```python
from build123d import *

# Parameters (mm, degrees)
SKETCH1_W           = 540
SKETCH1_H           = 540
BOSS_EXTRUDE1_DEPTH = 5
SKETCH2_W           = 20
SKETCH2_H           = 20
CUT_EXTRUDE1_DEPTH  = 5
CHAMFER1_SIZE       = 2
CHAMFER2_SIZE       = 0.5
SKETCH3_W           = 200
SKETCH3_H           = 77.416612185
CUT_EXTRUDE2_DEPTH  = 10
CIRPATTERN1_COUNT   = 4


with BuildPart() as part:
    # Sketch1 → Boss-Extrude1 (new body)
    with BuildSketch(Plane.XY):
        with Locations((270, 270)):
            Rectangle(SKETCH1_W, SKETCH1_H)
    extrude(amount=BOSS_EXTRUDE1_DEPTH)

    # Sketch2 → Cut-Extrude1 (cut)
    with BuildSketch(Plane.XY.offset(5)):
        with Locations((10, 530)):
            Rectangle(SKETCH2_W, SKETCH2_H)
        with Locations((530, 530)):
            Rectangle(SKETCH2_W, SKETCH2_H)
        with Locations((530, 10)):
            Rectangle(SKETCH2_W, SKETCH2_H)
        with Locations((10, 10)):
            Rectangle(SKETCH2_W, SKETCH2_H)
    extrude(amount=-CUT_EXTRUDE1_DEPTH, mode=Mode.SUBTRACT)

    # Chamfer1
    chamfer1_edges = [part.edges().sort_by_distance(p)[0] for p in [
        (0, 20, 2.5),
        (20, 0, 2.5),
        (540, 20, 2.5),
        (520, 0, 2.5),
        (540, 520, 2.5),
        (520, 540, 2.5),
        (0, 520, 2.5),
        (20, 540, 2.5),
    ]]
    chamfer(chamfer1_edges, length=CHAMFER1_SIZE)

    # Chamfer2
    chamfer2_edges = [part.edges().sort_by_distance(p)[0] for p in [
        (11, 20, 0),
        (11, 20, 5),
        (520, 11, 0),
        (520, 11, 5),
        (529, 520, 0),
        (529, 520, 5),
        (20, 529, 0),
        (20, 529, 5),
        (11, 520, 5),
        (11, 520, 0),
        (0, 270, 5),
        (20, 11, 5),
        (270, 0, 5),
        (529, 20, 5),
        (540, 270, 5),
        (520, 529, 5),
        (270, 540, 5),
        (519, 1, 5),
        (539, 21, 5),
        (1, 21, 5),
        (21, 1, 5),
        (539, 519, 5),
        (519, 539, 5),
        (21, 539, 5),
        (1, 519, 5),
        (0, 270, 0),
        (270, 540, 0),
        (520, 529, 0),
        (540, 270, 0),
        (529, 20, 0),
        (270, 0, 0),
        (20, 11, 0),
        (519, 1, 0),
        (539, 21, 0),
        (1, 21, 0),
        (21, 1, 0),
        (539, 519, 0),
        (519, 539, 0),
        (21, 539, 0),
        (1, 519, 0),
    ]]
    chamfer(chamfer2_edges, length=CHAMFER2_SIZE)

    # Sketch3 → Cut-Extrude2 (cut)
    with BuildSketch(Plane.XY.offset(5)):
        with Locations((270, 558.708306093)):
            Rectangle(SKETCH3_W, SKETCH3_H)
    cut_extrude2 = extrude(amount=-CUT_EXTRUDE2_DEPTH, mode=Mode.SUBTRACT)

    # CirPattern1: Cut-Extrude2 ×4 about axis
    cirpattern1_axis = Axis((270, 270, 0), (0, 0, 1))
    for i in range(1, CIRPATTERN1_COUNT):
        add(cut_extrude2.rotate(cirpattern1_axis, i * 360 / CIRPATTERN1_COUNT), mode=Mode.SUBTRACT)


solid = part.part
```
Source: CAD feature listing. Evaluate the final solid. Frame: model axes, mm. Round coordinates to 2 decimals unless told otherwise and drop trailing zeros. Write each loop counter-clockwise with the first axis right and the second up, starting at its lowest first coordinate (ties: lowest second). Pieces come first, ordered by that corner, then holes. Notation, with made-up numbers: M -27,-23 L -4,-23 A26 cw -4,13 Z; hole C -12,1.25 d5. An arc over 180 degrees is marked long. Use CSV: the item, a comma, the result in double quotes. Start each with the question number.
Q1. Cut plane A-A on y = 351. Output: boundary loops of the cut face in (x, z), plus the area to 3 significant figures.
Q2. Line query: line 1 (Y direction, x = 275.5, z = 4.3); line 2 (Y direction, x = 114.5, z = 4.7). Output: solid intervals per line, ascending. Write a range as from..to.
Q3. First-contact query: P1, Ø2.5, axis at y = 242, z = 3.5, coming from the -X side; P2, Ø1.2, axis at y = 9, z = 2, coming from the +X side; P3, Ø2, axis at x = 305.5, z = 1, coming from the +Y side. Flat tips, straight axial feed; report the tip coordinate or a pass-through.
Results found:
1,outline,"M 20,0 L 520,0 L 520,5 L 20,5 Z"
1,area,"2,500 mm^2"
2,line 1,"20..520"
2,line 2,"0.2..539.8"
3,P1,"x = 20"
3,P2,"x = 520"
3,P3,"y = 520"
